```python
from build123d import *

# Parameters (mm, degrees)
SKETCH1_W           = 25
SKETCH1_H           = 15
BOSS_EXTRUDE1_DEPTH = 27.5
BOSS_EXTRUDE1_TAPER = 3
FILLET1_R           = 1.5
SKETCH2_W           = 4
SKETCH2_H           = 4
BOSS_EXTRUDE2_DEPTH = 21
CUT_EXTRUDE1_DEPTH  = 1.75


with BuildPart() as part:
    # Sketch1 → Boss-Extrude1 (new body)
    with BuildSketch(Plane(origin=(0, 0, 0), x_dir=(1, 0, 0), z_dir=(0, 1, 0))):
        Rectangle(SKETCH1_W, SKETCH1_H)
    extrude(amount=BOSS_EXTRUDE1_DEPTH, taper=BOSS_EXTRUDE1_TAPER)

    # Fillet1
    fillet1_edges = [part.edges().sort_by_distance(p)[0] for p in [
        (-11.05878607, 27.5, 0),
        (0, 27.5, 6.05878607),
        (11.05878607, 27.5, 0),
        (0, 0, 7.5),
        (-12.5, 0, 0),
        (0, 0, -7.5),
        (12.5, 0, 0),
        (11.779393035, 13.75, 6.779393035),
        (-11.779393035, 13.75, 6.779393035),
        (-11.779393035, 13.75, -6.779393035),
        (11.779393035, 13.75, -6.779393035),
        (0, 27.5, -6.05878607),
    ]]
    fillet(fillet1_edges, radius=FILLET1_R)

    # Sketch2 → Boss-Extrude2 (add)
    with BuildSketch(Plane(origin=(0, 0, 0), x_dir=(-1, 0, 0), z_dir=(0, -1, 0))):
        Rectangle(SKETCH2_W, SKETCH2_H)
    extrude(amount=BOSS_EXTRUDE2_DEPTH)

    # Sketch3 → Cut-Extrude1 (cut, symmetric)
    with BuildSketch(Plane.XY):
        with BuildLine():
            Line((-9.63533922, 27.5), (9.63533922, 27.5))
            ThreePointArc((9.63533922, 27.5), (10.667871083, 27.088061557), (11.133283522, 26.078503934))
            Line((11.133283522, 26.078503934), (10.633968754, 26.052335956))
            ThreePointArc((10.633968754, 26.052335956), (10.323693795, 26.725374371), (9.63533922, 27))
            Line((9.63533922, 27), (-9.63533922, 27))
            ThreePointArc((-9.63533922, 27), (-10.323693795, 26.725374371), (-10.633968754, 26.052335956))
            Line((-10.633968754, 26.052335956), (-11.133283522, 26.078503934))
            ThreePointArc((-11.133283522, 26.078503934), (-10.667871083, 27.088061557), (-9.63533922, 27.5))
        make_face()
    extrude(amount=CUT_EXTRUDE1_DEPTH, both=True, mode=Mode.SUBTRACT)


solid = part.part
```
The listing builds one solid part. Answer for the finished solid, in the listing's coordinates (mm). A direction names the side the tool comes from. Coordinates: 2 decimals unless noted, no trailing zeros. Loops run counter-clockwise (first coordinate to the right, second up) from the corner with the lowest first, then second, coordinate; pieces in that order, holes last. Notation, with made-up numbers: (61, 16.5) - (117, 16.5) arc R16 ccw to (117, 24.5) - close; hole circle Ø8 at (61, 4). An arc over 180 degrees is marked (long way). Use a Markdown table: item, result. Add a question column.
1) Given pin 1 (1.6 mm diameter, centred on x = -4.5, y = 27, fed in from -Z); pin 2 (1.2 mm diameter, centred on y = -9.5, z = 0, fed in from +X); pin 3 (3 mm diameter, centred on y = -15.5, z = 0, fed in from -X), each flat-ended and moving along its own axis, determine where each tip first touches the part or whether it passes through.
2) The mould has two halves that part along Z. Classify faces 5 (the flat face through (0.1, 27.3, -1.75)), 6 (the flat face through (0, 27.5, -3)), 7 (the flat face through (0, -10, -2)): released by +Z, released by -Z, zero draft, split by the parting line, or undercut.
3) For faces 1 (the flat face through (2, -10, 0)), 2 (the flat face through (0, -10, 2)), 3 (the flat face through (0, 27, 0)), 4 (the flat face through (-2, -10, 0)), determine the directions among +Z, -Z, +X, -X, +Y, -Y from which every point of the face is accessible in a straight line to the end or side of a thin tool.
4) The part is cut by section A-A, the plane y = -18. Give the vertices of the cut face in (x, z), and give its area (3 significant figures).
5) Find the intervals of material crossed by line 1 (Y direction, x = -4, z = 3); line 2 (Z direction, x = 1, y = 26); line 3 (X direction, y = -11.5, z = 1.25), in increasing order.
Here are the results:
| question | item | result |
|---|---|---|
| 1 | pin 1 | stops at z = -6.12 |
| 1 | pin 2 | stops at x = 2 |
| 1 | pin 3 | stops at x = -2 |
| 2 | face 5 | undercut |
| 2 | face 6 | zero draft |
| 2 | face 7 | released by -Z |
| 3 | face 1 | +Z, -Z, +X, -Y |
| 3 | face 2 | +Z, +X, -X, -Y |
| 3 | face 3 | +X, -X, +Y |
| 3 | face 4 | +Z, -Z, -X, -Y |
| 4 | outline | (-2, -2) - (2, -2) - (2, 2) - (-2, 2) - close |
| 4 | area | 16.0 mm^2 |
| 5 | line 1 | y = 0 to 27.5 |
| 5 | line 2 | z = -6.14 to 6.14 |
| 5 | line 3 | x = -2 to 2 |
